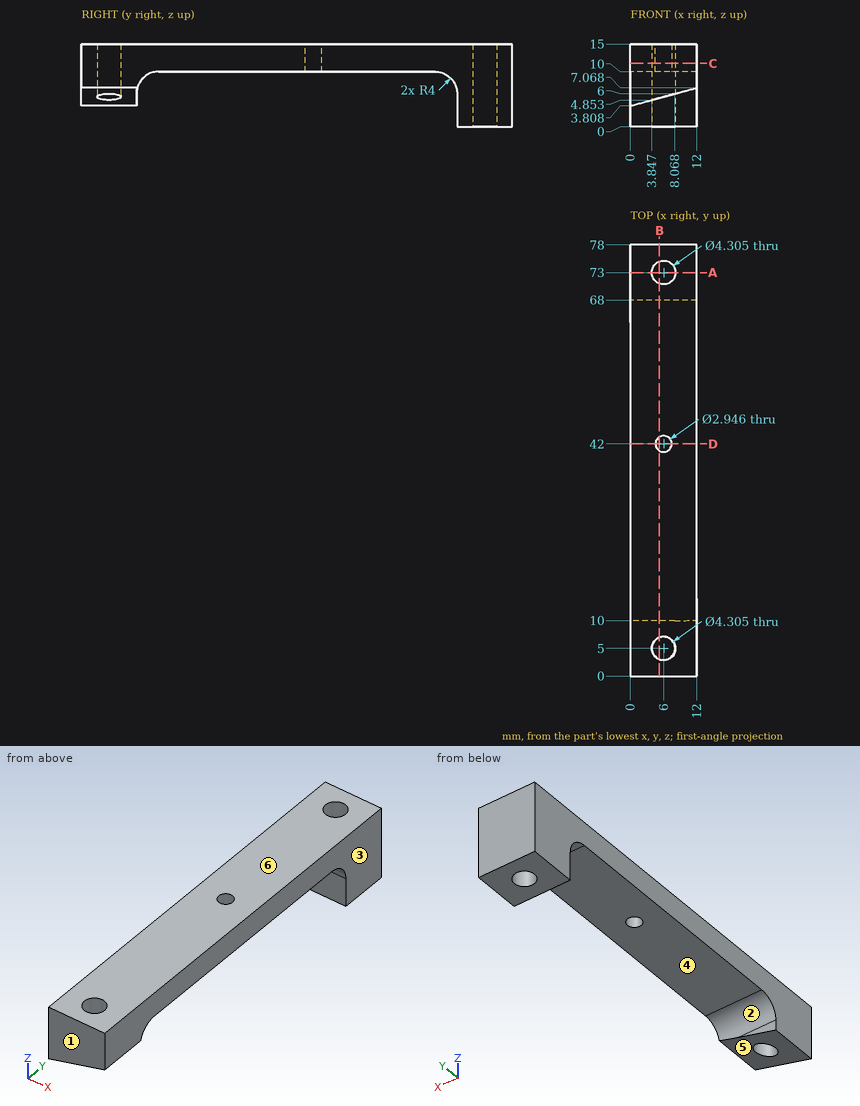
Check sheet for the drawn part. Datum: minimum x, y, z corner. Units: mm. A direction names the side the tool comes from. Give positions to 0.01 mm unless a question says otherwise; leave off trailing zeros. Order: outer loops, then holes, each group sorted by start corner. A loop starts at its lowest first (then second) coordinate and runs counter-clockwise, first axis right, second up. Notation, with made-up numbers: (78.25, -27) -> (97.25, -27) arc R15 ccw to (97.25, -20) -> close; hole circle Ø7 at (37.25, 41.25). An arc over 180 degrees is marked (long way). Return JSON: item names as keys, results as strings.
1. Cross-section at D-D, the plane y = 42. Record the cut outline in (x, z).
From the geometry:
{"outline": "(0, 10) -> (4.53, 10) -> (4.53, 15) -> (0, 15) -> close; (7.47, 10) -> (12, 10) -> (12, 15) -> (7.47, 15) -> close"}
2. Material ranges on probe 1 along Y at (x, z) = (6, 12.4); probe 2 along Y at (x, z) = (7.75, 11.75) (1 decimal); probe 3 along Z at (x, y) = (3.5, 36.5), recorded low to high. Write a range as [from, to].
From the geometry:
{"probe 1": "[0, 2.85], [7.15, 40.53], [43.47, 70.85], [75.15, 78]", "probe 2": "[0, 3.7], [6.3, 71.7], [74.3, 78]", "probe 3": "[10, 15]"}
3. Cross-section at B-B, the plane x = 5.25. Record the cut outline in (y, z) (1 decimal).
From the geometry:
{"outline": "(0, 5.2) -> (3, 5.2) -> (3, 15) -> (0, 15) -> close; (7, 5.2) -> (10, 5.2) -> (10, 6) arc R4 cw to (14, 10) -> (40.7, 10) -> (40.7, 15) -> (7, 15) -> close; (43.3, 10) -> (64, 10) arc R4 cw to (68, 6) -> (68, 0) -> (71, 0) -> (71, 15) -> (43.3, 15) -> close; (75, 0) -> (78, 0) -> (78, 15) -> (75, 15) -> close"}
4. Mould release check, pull along Y, two halves, no side actions. Record for the marked faces 1, 2 and 3: +Y half, -Y half, draft (parallel to the pull), parting line (faces both ways), or undercut.
From the geometry:
{"face 1": "-Y half", "face 2": "undercut", "face 3": "draft"}
5. Cross-section at A-A, the plane y = 73. Record the cut outline in (x, z).
From the geometry:
{"outline": "(0, 0) -> (3.85, 0) -> (3.85, 15) -> (0, 15) -> close; (8.15, 0) -> (12, 0) -> (12, 15) -> (8.15, 15) -> close"}
6. Set-up check for the marked faces 4, 5 and 6: record each of +Z, -Z, +X, -X, +Y, -Y from which the full face is reachable in a straight line by a thin tool's end or side.
From the geometry:
{"face 4": "-Z, +X, -X", "face 5": "-Z, +X, -Y", "face 6": "+Z, +X, -X, +Y, -Y"}
7. Cross-section at C-C, the plane z = 11.5. Record the cut outline in (x, y) (1 decimal).
From the geometry:
{"outline": "(0, 0) -> (12, 0) -> (12, 78) -> (0, 78) -> close; hole circle Ø4.3 at (6, 5); hole circle Ø4.3 at (6, 73); hole circle Ø2.9 at (6, 42)"}
8. Go/stop test with flat-tipped pins: P1, Ø5, axis at x = 7, y = 47, coming from the -Z side; P2, Ø2, axis at y = 45, z = 8, coming from the -X side. Record where each tip stops, or that it passes through.
From the geometry:
{"P1": "z = 10", "P2": "through"}
